from build123d import *

# Parameters (mm, degrees)
BOX007_W          = 39
BOX007_H          = 22
BOX007_DEPTH      = 1.6
BOX006_W          = 38.6
BOX006_H          = 20.6
BOX006_DEPTH      = 6.6
BOX_W             = 40
BOX_H             = 24
BOX_DEPTH         = 8.1
FILLET_R          = 1
CYLINDER001_R     = 1.9
CYLINDER001_DEPTH = 10
ARRAY002_Y_COUNT  = 2
ARRAY002_Y_PITCH  = 40
BOX005_W          = 9.8
BOX005_H          = 50
BOX005_DEPTH      = 3
FILLET002_R       = 4


with BuildPart() as pcb_extract_cube:
    # Box007 → Box007 (new body)
    with BuildSketch(Plane(origin=(1, 1, 3.5), x_dir=(1, 0, 0), z_dir=(0, 0, 1))):
        with Locations((19.5, 11)):
            Rectangle(BOX007_W, BOX007_H)
    extrude(amount=BOX007_DEPTH)


with BuildPart() as extract_fusion:
    # Box006 → Box006 (new body)
    with BuildSketch(Plane(origin=(1.7, 1.7, 1.5), x_dir=(1, 0, 0), z_dir=(0, 0, 1))):
        with Locations((19.3, 10.3)):
            Rectangle(BOX006_W, BOX006_H)
    extrude(amount=BOX006_DEPTH)

    # Fusion: union pcb extract cube
    add(pcb_extract_cube.part)


with BuildPart() as external_fillet:
    # Box → Box (new body)
    with BuildSketch(Plane.XY):
        with Locations((20, 12)):
            Rectangle(BOX_W, BOX_H)
    extrude(amount=BOX_DEPTH)

    # Fillet
    fillet_edges = [external_fillet.edges().sort_by_distance(p)[0] for p in [
        (0, 0, 4.05),
        (0, 24, 4.05),
        (40, 0, 4.05),
        (40, 24, 4.05),
    ]]
    fillet(fillet_edges, radius=FILLET_R)


with BuildPart() as attach_hole_array:
    # Cylinder001 → Cylinder001 (new body)
    with BuildSketch(Plane(origin=(5, 4.9, 0), x_dir=(1, 0, 0), z_dir=(0, 0, 1))):
        Circle(CYLINDER001_R)
    extrude(amount=CYLINDER001_DEPTH)

    # Array002 Y: attach hole array ×2


with BuildPart() as attach_hole_array_1:
    add(attach_hole_array.part)
    with Locations(*[(0, i * ARRAY002_Y_PITCH, 0) for i in range(1, ARRAY002_Y_COUNT)]):
        add(attach_hole_array.part)


with BuildPart() as obj1:
    # Box005 → Box005 (new body)
    with BuildSketch(Plane.XY):
        with Locations((4.9, 25)):
            Rectangle(BOX005_W, BOX005_H)
    extrude(amount=BOX005_DEPTH)

    # Fillet002
    fillet002_edges = [obj1.edges().sort_by_distance(p)[0] for p in [
        (0, 0, 1.5),
        (0, 50, 1.5),
        (9.8, 0, 1.5),
        (9.8, 50, 1.5),
    ]]
    fillet(fillet002_edges, radius=FILLET002_R)

    # Cut002: cut attach hole array
    add(attach_hole_array_1.part, mode=Mode.SUBTRACT)


with BuildPart() as obj1_1:
    # Cut002 placement: moved
    add(obj1.part.moved(Location((15.6, -13, 0))))

    # Fusion001: union external fillet
    add(external_fillet.part)

    # Cut: cut extract fusion
    add(extract_fusion.part, mode=Mode.SUBTRACT)


solid = obj1_1.part
Design review of the part built by this model. Coordinates are the model's own, in mm. A direction names the side the tool comes from. Round coordinates to 2 decimals unless told otherwise and drop trailing zeros. Loops run counter-clockwise (first coordinate to the right, second up) from the corner with the lowest first, then second, coordinate; pieces in that order, holes last. Notation, with made-up numbers: (73.5, 55) - (97.5, 55) arc R24 cw to (97.5, 89) - close; hole circle Ø10 at (70, 10.5). An arc over 180 degrees is marked (long way). One line per question, with ' | ' between items.
1. Draft analysis for pull direction Y (two halves, no side actions). For faces 4 (the face through (15.6, 28, 1)), 5 (the face through (20, 23, 4)), 6 (the face through (16.741, 35.797, 1.521)), state which applies: released by +Y, released by -Y, zero draft, split by the parting line, or undercut.
Results are:
face 4: zero draft | face 5: undercut | face 6: released by +Y
2. For L1, parallel to Y at x = 20.6, z = 1.4; L2, parallel to Y at x = 20.6, z = 2.3; L3, parallel to Z at x = 7, y = 1.5, list the stretches that pass through material, from the lowest coordinate up. Write a range as [from, to].
Results are:
L1: y = [-13, -10], [-6.2, 30], [33.8, 37] | L2: y = [-13, -10], [-6.2, 1.7], [22.3, 30], [33.8, 37] | L3: z = [0, 3.5], [5.1, 8.1]
3. We need section C-C, the plane z = 2.25. State the section outline as (x, y) points, and give its area (3 significant figures).
Results are:
outline: (0, 1) arc R1 ccw to (1, 0) - (15.6, 0) - (15.6, -9) arc R4 ccw to (19.6, -13) - (21.4, -13) arc R4 ccw to (25.4, -9) - (25.4, 0) - (39, 0) arc R1 ccw to (40, 1) - (40, 1.7) - (1.7, 1.7) - (1.7, 22.3) - (40, 22.3) - (40, 23) arc R1 ccw to (39, 24) - (25.4, 24) - (25.4, 33) arc R4 ccw to (21.4, 37) - (19.6, 37) arc R4 ccw to (15.6, 33) - (15.6, 24) - (1, 24) arc R1 ccw to (0, 23) - close; hole circle Ø3.8 at (20.6, -8.1); hole circle Ø3.8 at (20.6, 31.9) | area: 389 mm²
4. Clearance check with flat-ended pins moving along their axes: P1, Ø2, axis at x = 33.5, z = 2, coming from the +Y side; P2, Ø2, axis at x = 8, z = 4.5, coming from the -Y side; P3, Ø2.5, axis at y = 27, z = 2, coming from the -X side. State where each tip first meets the part, or that it passes through.
Results are:
P1: stops at y = 24 | P2: stops at y = 0 | P3: stops at x = 15.6
5. We need section A-A, the plane y = -8.1. State the section outline as (x, z) points.
Results are:
outline: (15.6, 0) - (18.7, 0) - (18.7, 3) - (15.6, 3) - close; (22.5, 0) - (25.4, 0) - (25.4, 3) - (22.5, 3) - close
6. For faces 1 (the face through (14.6, 1.5, 3.5)), 2 (the face through (1.7, 12, 2)), 3 (the face through (15.6, -5, 1)), list the 3-axis set-ups (+Z, -Z, +X, -X, +Y, -Y) from which the entire face can be reached by the end or side of a thin tool; tool diameter is ignored.
Results are:
face 1: +X | face 2: +Z, +X | face 3: +Z, -Z, -X, -Y
7. We need section B-B, the plane x = 20.6. State the section outline as (y, z) points.
Results are:
outline: (-13, 0) - (-10, 0) - (-10, 3) - (-13, 3) - close; (-6.2, 0) - (30, 0) - (30, 3) - (24, 3) - (24, 8.1) - (22.3, 8.1) - (22.3, 5.1) - (23, 5.1) - (23, 3.5) - (22.3, 3.5) - (22.3, 1.5) - (1.7, 1.5) - (1.7, 3.5) - (1, 3.5) - (1, 5.1) - (1.7, 5.1) - (1.7, 8.1) - (0, 8.1) - (0, 3) - (-6.2, 3) - close; (33.8, 0) - (37, 0) - (37, 3) - (33.8, 3) - close
8. We need section D-D, the plane y = 15. State the section outline as (x, z) points.
Results are:
outline: (0, 0) - (40, 0) - (40, 1.5) - (1.7, 1.5) - (1.7, 3.5) - (1, 3.5) - (1, 5.1) - (1.7, 5.1) - (1.7, 8.1) - (0, 8.1) - close
